```python
from build123d import *

# Parameters (mm, degrees)
SKETCH053_W     = 4
SKETCH053_H     = 27
PAD030_DEPTH    = 45.4
SKETCH054_R     = 1.5
POCKET022_DEPTH = 5
SKETCH055_R     = 2.75
POCKET023_DEPTH = 2.4
SKETCH056_W     = 35
SKETCH056_H     = 53.4
SKETCH056_W_2   = 27
SKETCH056_H_2   = 45.4
PAD031_DEPTH    = 8
SKETCH057_W     = 76
SKETCH057_H     = 44
SKETCH057_R     = 2
SKETCH057_W_2   = 30
SKETCH057_H_2   = 30
PAD032_DEPTH    = 4
SKETCH058_W     = 50
SKETCH058_H     = 12
POCKET024_DEPTH = 4


with BuildPart() as left001:
    # Sketch053 → Pad030 (new body)
    with BuildSketch(Plane.XY):
        Rectangle(SKETCH053_W, SKETCH053_H)
    extrude(amount=PAD030_DEPTH)

    # Sketch054 (on Face2 of Pad030) → Pocket022 (cut)
    with BuildSketch(Plane.YZ.offset(2)):
        with Locations((-10, 32.7)):
            Circle(SKETCH054_R)
        with Locations((10, 32.7)):
            Circle(SKETCH054_R)
        with Locations((10, 12.7)):
            Circle(SKETCH054_R)
        with Locations((-10, 12.7)):
            Circle(SKETCH054_R)
    extrude(amount=-POCKET022_DEPTH, mode=Mode.SUBTRACT)

    # Sketch055 (on Face2 of Pad030) → Pocket023 (cut)
    with BuildSketch(Plane.YZ.offset(2)):
        with Locations((-10, 32.7)):
            Circle(SKETCH055_R)
        with Locations((10, 32.7)):
            Circle(SKETCH055_R)
        with Locations((10, 12.7)):
            Circle(SKETCH055_R)
        with Locations((-10, 12.7)):
            Circle(SKETCH055_R)
    extrude(amount=-POCKET023_DEPTH, mode=Mode.SUBTRACT)

    # Sketch056 (on Face3 of Pocket023) → Pad031 (join)
    with BuildSketch(Plane.YZ.offset(2)):
        with Locations((0, 22.7)):
            Rectangle(SKETCH056_W, SKETCH056_H)
        with Locations((0, 22.7)):
            Rectangle(SKETCH056_W_2, SKETCH056_H_2, mode=Mode.SUBTRACT)
    extrude(amount=-PAD031_DEPTH)

    # Sketch057 (on Face23 of Pad031) → Pad032 (join)
    with BuildSketch(Plane.YZ.offset(2)):
        with Locations((0, 22.7)):
            Rectangle(SKETCH057_W, SKETCH057_H)
        with Locations((-32, 38.7)):
            Circle(SKETCH057_R, mode=Mode.SUBTRACT)
        with Locations((32, 38.7)):
            Circle(SKETCH057_R, mode=Mode.SUBTRACT)
        with Locations((32, 6.7)):
            Circle(SKETCH057_R, mode=Mode.SUBTRACT)
        with Locations((-32, 6.7)):
            Circle(SKETCH057_R, mode=Mode.SUBTRACT)
        with Locations((-24, 38.7)):
            Circle(SKETCH057_R, mode=Mode.SUBTRACT)
        with Locations((24, 38.7)):
            Circle(SKETCH057_R, mode=Mode.SUBTRACT)
        with Locations((24, 6.7)):
            Circle(SKETCH057_R, mode=Mode.SUBTRACT)
        with Locations((-24, 6.7)):
            Circle(SKETCH057_R, mode=Mode.SUBTRACT)
        with Locations((0, 22.7)):
            Rectangle(SKETCH057_W_2, SKETCH057_H_2, mode=Mode.SUBTRACT)
    extrude(amount=-PAD032_DEPTH)

    # Sketch058 (on Face4 of Pad032) → Pocket024 (cut)
    with BuildSketch(Plane(origin=(-6, 0, 0), x_dir=(0, -1, 0), z_dir=(-1, 0, 0))):
        with Locations((0, 39.4)):
            Rectangle(SKETCH058_W, SKETCH058_H)
        with Locations((0, 6)):
            Rectangle(SKETCH058_W, SKETCH058_H)
    extrude(amount=-POCKET024_DEPTH, mode=Mode.SUBTRACT)


with BuildPart() as left001_1:
    # Body017 placement: moved
    add(left001.part.moved(Location((-98, -275.5, -9.2))))


with BuildPart() as right001:
    # Part__Mirroring006: instance of Left001
    add(left001_1.part.mirror(Plane(origin=(0, 0, 0), x_dir=(0, -1, 0), z_dir=(1, 0, 0))))


solid = right001.part
```
Could you check a few things on this model? Use its own coordinates, in mm. A direction names the side the tool comes from. Round coordinates to 2 decimals unless told otherwise and drop trailing zeros. Loops run counter-clockwise (first coordinate to the right, second up) from the corner with the lowest first, then second, coordinate; pieces in that order, holes last. Notation, with made-up numbers: M 49.25,-7.5 L 90.25,-7.5 A14 cw 90.25,16.5 Z; hole C 25,9.5 d1. An arc over 180 degrees is marked long. Answer as CSV lines item,"result".
1) For pin 1 Ø4 at (x, z) = (100, -11) entering from -Y; pin 2 Ø3 at (y, z) = (-243.5, -2.5) entering from +X; pin 3 Ø1.2 at (x, y) = (97.5, -304) entering from +Z; pin 4 Ø5 at (y, z) = (-265.5, 23.5) entering from +X, each with a flat end and sliding along its axis, tell me the tip position at first contact or that it passes through.
From the geometry:
pin 1,"y = -293"
pin 2,"through"
pin 3,"z = 35.5"
pin 4,"x = 100"
2) Imagine slicing it at C-C on z = 8.5. List the corners of the cut face in (x, y) for me.
From the geometry:
outline,"M 96,-313.5 L 100,-313.5 L 100,-293 L 104,-293 L 104,-289 L 100,-289 L 100,-262 L 104,-262 L 104,-258 L 100,-258 L 100,-237.5 L 96,-237.5 Z"
3) Imagine slicing it at D-D on y = -285.5. List the corners of the cut face in (x, z) for me, and give its area (3 significant figures).
From the geometry:
outline,"M 96,-13.2 L 104,-13.2 L 104,-9.2 L 100,-9.2 L 100,2 L 98.4,2 L 98.4,0.75 L 96,0.75 Z; M 96,6.25 L 98.4,6.25 L 98.4,5 L 100,5 L 100,22 L 98.4,22 L 98.4,20.75 L 96,20.75 Z; M 96,26.25 L 98.4,26.25 L 98.4,25 L 100,25 L 100,36.2 L 104,36.2 L 104,40.2 L 96,40.2 Z"
area,"210 mm^2"
4) If I drill on probe 1 along Z at (x, y) = (96.5, -265.5); probe 2 along Z at (x, y) = (97.4, -307.5); probe 3 along Z at (x, y) = (101.75, -263), over which ranges is the centre line in solid material (lowest first)?
From the geometry:
probe 1,"-13.2 to 0.75, 6.25 to 20.75, 26.25 to 40.2"
probe 2,"-8.5 to -4.5, -0.5 to 27.5, 31.5 to 35.5"
probe 3,"-13.2 to -9.2, 36.2 to 40.2"
5) Which directions (+Z, -Z, +X, -X, +Y, -Y) give clear straight access to the entire face, cutting with the end or side of a thin tool? Please do faces 1 (the flat face through (102, -258, 13)), 2 (the flat face through (102, -275, 36.2)), 3 (the cylindrical face through (97.18, -282.88, 4.33)), 4 (the flat face through (98, -248, -8.5)), 5 (the flat face through (104, -260, 14)).
From the geometry:
face 1,"+Z, -Z, +X, +Y"
face 2,"+X, +Y, -Y"
face 3,"-X"
face 4,"-Z, +X, -X, +Y"
face 5,"+Z, -Z, +X, +Y, -Y"
6) We'd pull the mould along Z, two halves only. Please class faces 6 (the cylindrical face through (97.972, -306.577, 27.726)), 7 (the flat face through (98, -248, 35.5)), 8 (the flat face through (100, -258, -11)), 9 (the flat face through (98, -303, -8.5)): released by +Z, released by -Z, zero draft, split by the parting line, or undercut.
From the geometry:
face 6,"undercut"
face 7,"released by +Z"
face 8,"zero draft"
face 9,"released by -Z"
7) Imagine slicing it at B-B on x = 97.25. Count the separate pieces of the cut face and the enclosed holes in it, and give its area (3 significant figures).
From the geometry:
separate pieces,"1"
enclosed holes,"12"
area,"3,480 mm^2"
8) Imagine slicing it at A-A on y = -299.5. List the corners of the cut face in (x, z) for me, and give its area (3 significant figures).
From the geometry:
outline,"M 96,-8.5 L 100,-8.5 L 100,-4.5 L 96,-4.5 Z; M 96,-0.5 L 100,-0.5 L 100,27.5 L 96,27.5 Z; M 96,31.5 L 100,31.5 L 100,35.5 L 96,35.5 Z"
area,"144 mm^2"
